The model under review builds one solid part; all positions refer to its coordinate system, in mm. Face numbers are marked on the shaded views. A direction names the side the tool comes from. Give positions to 0.01 mm unless a question says otherwise; leave off trailing zeros. Loops run counter-clockwise (first coordinate to the right, second up) from the corner with the lowest first, then second, coordinate; pieces in that order, holes last. Notation, with made-up numbers: M -9.75,7 L 15.25,7 A20 ccw 15.25,22 Z; hole C 59.5,-3 d9. An arc over 180 degrees is marked long. One line per item, written item: value. Start each with the question number.
Q1. We need section A-A on z = 4.25. Write out the cut boundary in (x, y), plus the area to 3 significant figures.
Q2. For the marked faces 3 and 4, list the 3-axis set-ups (+Z, -Z, +X, -X, +Y, -Y) from which the entire face can be reached by the end or side of a thin tool; tool diameter is ignored.
Q3. We need section B-B on x = 2. Write out the cut boundary in (y, z), plus the area to 3 significant figures.
Q4. Mouldability with a two-part tool opening along X and no side actions: class the marked faces 1 and 2 as released by +X, released by -X, zero draft, split by the parting line, or undercut.
Q5. For pin 1 (1.8 mm diameter, centred on x = 6, y = 0, fed in from +Z); pin 2 (2 mm diameter, centred on x = -6.5, z = 1, fed in from +Y); pin 3 (1.6 mm diameter, centred on x = -3, z = 0.5, fed in from -Y), all flat-tipped, find the tip position at first contact; note any pin that passes through.
Q6. To check wall thickness, follow line 1 along X through (y, z) = (0, 3); line 2 along X through (y, z) = (2.2, 3.5); line 3 along Z through (x, y) = (21.5, 0). State the ranges of each line that lie inside material, in increasing order. Write a range as from..to.
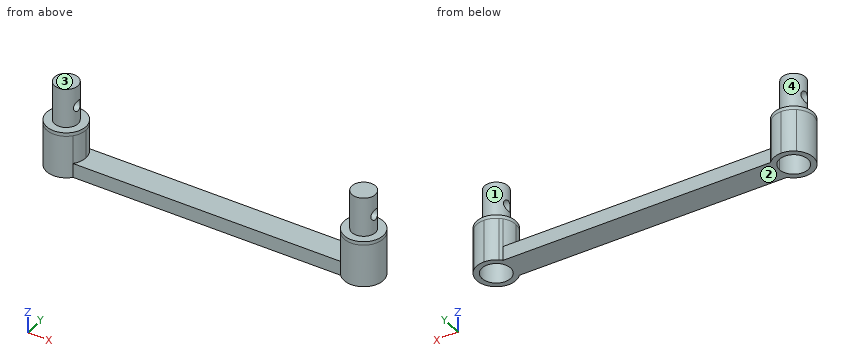
```python
from build123d import *

# Parameters (mm, degrees)
F1_DEPTH = 6
F2_DEPTH = 2
F3_R     = 2.75
F3_R_2   = 2
F4_DEPTH = 0.5
F5_R     = 1.65
F6_DEPTH = 5.5
F8_R     = 0.75
F9_DEPTH = 24.501


with BuildPart() as f1:
    # F0 (on Top) → F1 (new body)
    with BuildSketch(Plane.XY):
        with BuildLine():
            Line((-18.75, 0), (-18, 0))
            ThreePointArc((-18, 0), (-18.1731878907, 0.9604891218), (-18.6709377114, 1.8))
            ThreePointArc((-18.6709377114, 1.8), (-18.8287396862, 1.967551475), (-19, 2.1213203436))
            ThreePointArc((-19, 2.1213203436), (-19.8202502877, 2.5880621075), (-20.75, 2.75))
            Line((-20.75, 2.75), (-20.75, 2))
            ThreePointArc((-20.75, 2), (-19.3357864376, 1.4142135624), (-18.75, 0))
        make_face()
        with BuildLine():
            ThreePointArc((-18.6709377114, -1.8), (-18.1731878907, -0.9604891218), (-18, 0))
            Line((-18, 0), (-18.75, 0))
            ThreePointArc((-18.75, 0), (-22.1642135624, -1.4142135624), (-20.75, 2))
            Line((-20.75, 2), (-20.75, 2.75))
            ThreePointArc((-20.75, 2.75), (-21.6797497123, 2.5880621075), (-22.5, 2.1213203436))
            ThreePointArc((-22.5, 2.1213203436), (-22.717551475, -1.9212603138), (-18.6709377114, -1.8))
        make_face()
    extrude(amount=F1_DEPTH)

    # F0 (on Top) → F2 (join)
    with BuildSketch(Plane.XY):
        with BuildLine():
            Line((-18, 0), (0, 0))
            Line((0, 0), (0, 1.8))
            Line((0, 1.8), (-18.6709377114, 1.8))
            ThreePointArc((-18.6709377114, 1.8), (-18.1731878907, 0.9604891218), (-18, 0))
        make_face()
        with BuildLine():
            Line((0, -1.8), (0, 0))
            Line((0, 0), (-18, 0))
            ThreePointArc((-18, 0), (-18.1731878907, -0.9604891218), (-18.6709377114, -1.8))
            Line((-18.6709377114, -1.8), (0, -1.8))
        make_face()
    extrude(amount=F2_DEPTH)

    # F3 (on face) → F4 (join)
    with BuildSketch(Plane.XY.offset(6)):
        with Locations((-20.75, 0)):
            Circle(F3_R)
        with Locations((-20.75, 0)):
            Circle(F3_R_2, mode=Mode.SUBTRACT)
        with Locations((-20.75, 0)):
            Circle(F3_R_2)
    extrude(amount=F4_DEPTH)

    # F5 (on face) → F6 (join)
    with BuildSketch(Plane.XY.offset(6.5)):
        with Locations((-20.75, 0)):
            Circle(F5_R)
    extrude(amount=F6_DEPTH)

    # F8 (on offset) → F9 (cut, through all)
    with BuildSketch(Plane.YZ.offset(1)):
        with Locations((0, 9.1180996969)):
            Circle(F8_R)
    extrude(amount=-F9_DEPTH, mode=Mode.SUBTRACT)

    # F10: F1 across plane


with BuildPart() as f1_1:
    add(f1.part)
    add(f1.part.mirror(Plane.YZ))


solid = f1_1.part
```
Solved:
1. outline: C -20.75,0 d5.5; C 20.75,0 d5.5; hole C -20.75,0 d4; hole C 20.75,0 d4
1. area: 22.4 mm2
2. face 3: +Z, +X, -X, +Y, -Y
2. face 4: +Z
3. outline: M -1.8,0 L 1.8,0 L 1.8,2 L -1.8,2 Z
3. area: 7.20 mm2
4. face 1: undercut
4. face 2: zero draft
5. pin 1: z = 2
5. pin 2: y = 1.8
5. pin 3: y = -1.8
6. line 1: -23.5..-22.75, -18.75..-18, 18..18.75, 22.75..23.5
6. line 2: -22.4..-19.1, 19.1..22.4
6. line 3: 6..8.37, 9.87..12
